from build123d import *

# Parameters (mm, degrees)
SKETCH1_W         = 90
SKETCH1_H         = 40
PLATE_DEPTH       = 8
SKETCH2_R         = 2.5
SKETCH2_R_2       = 2.55
SKETCH2_R_3       = 2.6
SKETCH2_R_4       = 2.65
SKETCH2_R_5       = 2.7
SKETCH2_R_6       = 5
SKETCH2_R_7       = 5.05
SKETCH2_R_8       = 5.1
SKETCH2_R_9       = 5.15
SKETCH2_R_10      = 5.2
TEST_HOLES_DEPTH  = 50.889878733
BED_CHAMFERS_SIZE = 0.5


with BuildPart() as part:
    # Sketch1 → Plate (new body)
    with BuildSketch(Plane(origin=(0, 0, 0), x_dir=(1, 0, 0), z_dir=(0, 1, 0))):
        Rectangle(SKETCH1_W, SKETCH1_H)
    extrude(amount=PLATE_DEPTH)

    # Sketch2 → Test holes (cut, through all)
    with BuildSketch(Plane(origin=(0, 8, 0), x_dir=(1, 0, 0), z_dir=(0, 1, 0))):
        with Locations(Location((-32, 10, 0), (0, 0, 270))):
            Circle(SKETCH2_R)
        with Locations(Location((-16, 10, 0), (0, 0, 270))):
            Circle(SKETCH2_R_2)
        with Locations(Location((0, 10, 0), (0, 0, 270))):
            Circle(SKETCH2_R_3)
        with Locations(Location((16, 10, 0), (0, 0, 270))):
            Circle(SKETCH2_R_4)
        with Locations(Location((32, 10, 0), (0, 0, 270))):
            Circle(SKETCH2_R_5)
        with Locations(Location((-32, -10, 0), (0, 0, 270))):
            Circle(SKETCH2_R_6)
        with Locations(Location((-16, -10, 0), (0, 0, 270))):
            Circle(SKETCH2_R_7)
        with Locations(Location((0, -10, 0), (0, 0, 270))):
            Circle(SKETCH2_R_8)
        with Locations(Location((16, -10, 0), (0, 0, 270))):
            Circle(SKETCH2_R_9)
        with Locations(Location((32, -10, 0), (0, 0, 270))):
            Circle(SKETCH2_R_10)
    extrude(amount=-TEST_HOLES_DEPTH, mode=Mode.SUBTRACT)

    # Bed chamfers
    bed_chamfers_edges = [part.edges().sort_by_distance(p)[0] for p in [
        (-16, 0, -12.55),
        (0, 0, -12.6),
        (16, 0, -12.65),
        (32, 0, -12.7),
        (-32, 0, 5),
        (-16, 0, 4.95),
        (0, 0, 4.9),
        (16, 0, 4.85),
        (32, 0, 4.8),
        (-32, 0, -12.5),
    ]]
    chamfer(bed_chamfers_edges, length=BED_CHAMFERS_SIZE)


solid = part.part
Model file for the job. Use its own axes, mm. Round coordinates to 2 decimals unless told otherwise and drop trailing zeros. Order: outer loops, then holes, each group sorted by start corner. A loop starts at its lowest first (then second) coordinate and runs counter-clockwise, first axis right, second up.
(1) Band-saw the part on D-D (x = 32). List the corners of the cut face in (y, z), then the cut area to 3 significant figures.
(2) Band-saw the part on A-A (z = -10). Give the number of separate pieces and of enclosed holes in the cut face, then the cut area to 3 significant figures.
(3) Drill centre lines: line 1 (X direction, y = 4.75, z = -10); line 2 (X direction, y = 2.25, z = 10); line 3 (Z direction, x = 14, y = 4.25). Where is each one in solid material? Low to high.
(4) Pull direction X, two halves, no side cores. Call faces 1 (the face through (-45, 4, 0)), 2 (the face through (10.972, 4.302, 8.884)), 3 (the face through (-1, 4, 20)), 4 (the face through (45, 4, 0)): released by +X, released by -X, zero draft, split by the parting line, or undercut.
(5) Band-saw the part on B-B (x = -16). List the corners of the cut face in (y, z), then the cut area to 3 significant figures.
Verdict:
1. outline: (0, -20) - (8, -20) - (8, -12.7) - (0.5, -12.7) - (0, -13.2) - close; (0, -6.8) - (0.5, -7.3) - (8, -7.3) - (8, 4.8) - (0.5, 4.8) - (0, 4.3) - close; (0, 15.7) - (0.5, 15.2) - (8, 15.2) - (8, 20) - (0, 20) - close
1. area: 193 mm2
2. separate pieces: 6
2. enclosed holes: 0
2. area: 511 mm2
3. line 1: x = -45 to -34.5, -29.5 to -18.55, -13.45 to -2.6, 2.6 to 13.35, 18.65 to 29.3, 34.7 to 45
3. line 2: x = -45 to -37, -27 to -21.05, -10.95 to -5.1, 5.1 to 10.85, 21.15 to 26.8, 37.2 to 45
3. line 3: z = -20 to -11.74, -8.26 to 5.25, 14.75 to 20
4. face 1: released by -X
4. face 2: undercut
4. face 3: zero draft
4. face 4: released by +X
5. outline: (0, -20) - (8, -20) - (8, -12.55) - (0.5, -12.55) - (0, -13.05) - close; (0, -6.95) - (0.5, -7.45) - (8, -7.45) - (8, 4.95) - (0.5, 4.95) - (0, 4.45) - close; (0, 15.55) - (0.5, 15.05) - (8, 15.05) - (8, 20) - (0, 20) - close
5. area: 198 mm2
